Source: CAD feature listing. Evaluate the final solid. Frame: model axes, mm. Round coordinates to 2 decimals unless told otherwise and drop trailing zeros. Order: outer loops, then holes, each group sorted by start corner. A loop starts at its lowest first (then second) coordinate and runs counter-clockwise, first axis right, second up. Notation, with made-up numbers: (87.25, -26) -> (94.25, -26) arc R32 cw to (94.25, 6) -> close; hole circle Ø11 at (28.5, 41). An arc over 180 degrees is marked (long way). Answer as CSV lines item,"result". Start each with the question number.
(1) Section query B-B (x = 10.5). Output: boundary loops of the cut face in (y, z).
(2) Section query C-C (z = 28). Output: boundary loops of the cut face in (x, y).
(3) Line query: line 1 along X through (y, z) = (-416, 51); line 2 along Z through (x, y) = (6, -1602); line 3 along Z through (x, y) = (8, -490). Output: solid intervals per line, ascending. Write a range as from..to.
(4) Section query A-A (y = -1676). Output: boundary loops of the cut face in (x, z).
(5) Contact query for flat-ended pins moving along their axis: P1, Ø10, axis at y = -614.5, z = 28, coming from the +X side; P2, Ø10, axis at y = -686, z = 59, coming from the +X side. Output: stop coordinate, or through.
```python
from build123d import *

# Parameters (mm, degrees)
F1_DEPTH = 2300


with BuildPart() as f1:
    # F0 (on Front) → F1 (new body)
    with BuildSketch(Plane.XZ):
        with BuildLine():
            Line((0, 45), (0, 0))
            Line((0, 0), (5, 0))
            ThreePointArc((5, 0), (15.419175, 21.436257), (19, 45))
            Line((19, 45), (0, 45))
        make_face()
        with BuildLine():
            Line((0, 90), (0, 45))
            Line((0, 45), (19, 45))
            ThreePointArc((19, 45), (15.419175, 68.563743), (5, 90))
            Line((5, 90), (0, 90))
        make_face()
    extrude(amount=F1_DEPTH)


solid = f1.part
```
Answer block:
1,outline,"(-2300, 9.28) -> (0, 9.28) -> (0, 80.72) -> (-2300, 80.72) -> close"
2,outline,"(0, -2300) -> (17.16, -2300) -> (17.16, 0) -> (0, 0) -> close"
3,line 1,"0..18.77"
3,line 2,"1.49..88.51"
3,line 3,"4.7..85.3"
4,outline,"(0, 0) -> (5, 0) arc R79.32 ccw to (19, 45) arc R79.32 ccw to (5, 90) -> (0, 90) -> close"
5,P1,"x = 18.09"
5,P2,"x = 18.49"
